Design review of the part shown in the three views and the two pictorial views. Dimensions are in mm from the part's minimum x, y and z. A direction names the side the tool comes from. Give positions to 0.01 mm unless a question says otherwise; leave off trailing zeros. Loops run counter-clockwise (first coordinate to the right, second up) from the corner with the lowest first, then second, coordinate; pieces in that order, holes last.
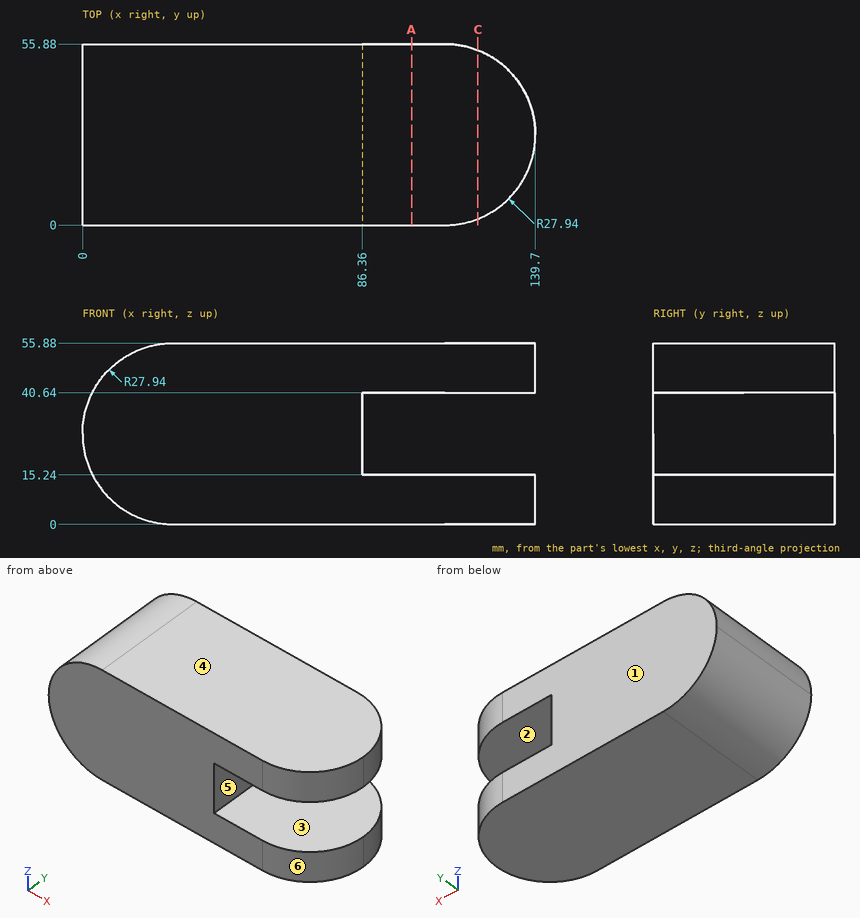
Q1. Consider section C-C on x = 122. Give the boundary of the cut face in (y, z), plus the area to 3 significant figures.
Answers:
outline: (1.94, 0) - (53.94, 0) - (53.94, 15.24) - (1.94, 15.24) - close; (1.94, 40.64) - (53.94, 40.64) - (53.94, 55.88) - (1.94, 55.88) - close
area: 1,580 mm2
Q2. Machinability: for the marked faces 5 and 6, which of the approach directions +Z, -Z, +X, -X, +Y, -Y give a long, thin tool a straight path to every point of the face, cutting with its end or side? Answer none if there is none.
Answers:
face 5: +X, +Y, -Y
face 6: +Z, -Z, +X, -Y
Q3. For pin 1 Ø1.5 at (x, z) = (115, 13.5) entering from +Y; pin 2 Ø1.5 at (y, z) = (33.5, 29.5) entering from +X; pin 3 Ø4 at (y, z) = (11.5, 39.5) entering from +X, all flat-tipped, find the tip position at first contact; note any pin that passes through.
Answers:
pin 1: stops at y = 55.77
pin 2: stops at x = 86.36
pin 3: stops at x = 135.46
Q4. For probe 1 along Z at (x, y) = (92, 27); probe 2 along X at (y, z) = (27, 28); probe 3 along X at (y, z) = (44.5, 37), list the stretches that pass through material, from the lowest coordinate up.
Answers:
probe 1: z = 0 to 15.24, 40.64 to 55.88
probe 2: x = 0 to 86.36
probe 3: x = 1.51 to 86.36
Q5. Consider section A-A on x = 101.5. Give the boundary of the cut face in (y, z), plus the area to 3 significant figures.
Answers:
outline: (0, 0) - (55.88, 0) - (55.88, 15.24) - (0, 15.24) - close; (0, 40.64) - (55.88, 40.64) - (55.88, 55.88) - (0, 55.88) - close
area: 1,700 mm2
Q6. Mouldability with a two-part tool opening along Z and no side actions: class the marked faces 1, 2, 3 and 4 as +Z half, -Z half, draft (parallel to the pull), parting line (faces both ways), or undercut.
Answers:
face 1: draft
face 2: undercut
face 3: undercut
face 4: +Z half
